Could you check a few things on this model? Use its own coordinates, in mm. A direction names the side the tool comes from. Coordinates: 2 decimals unless noted, no trailing zeros. Loops run counter-clockwise (first coordinate to the right, second up) from the corner with the lowest first, then second, coordinate; pieces in that order, holes last. Notation, with made-up numbers: (80.5, -25.75) - (120.5, -25.75) arc R22 ccw to (120.5, -9.75) - close; hole circle Ø1 at (57, -39). An arc over 180 degrees is marked (long way). One line per item, written item: value. Start each with the question number.
(1) If we section it at A-A on x = 0: Write out the boundary of the cut face in (y, z), then the cut area to 3 significant figures.
(2) If we section it at D-D on z = 15: Write out the boundary of the cut face in (x, y), then the cut area to 3 significant figures.
(3) If we mould it in two halves opening along Y, with no side actions, what happens to faces 4 (the face through (12.932, -5.362, 11.479)), 5 (the face through (-9.5, 0.07, 11.48)), 6 (the face through (2, 5, 39))? For each: pulls with the +Y half, pulls with the -Y half, needs draft (parallel to the pull), parting line crosses it, or undercut.
(4) I'm going to push flat-ended pins straight in: P1, Ø8, axis at x = -5.5, z = 11, coming from the +Y side; P2, Ø5, axis at x = -3.5, z = 8, coming from the +Y side; P3, Ø2, axis at y = 1, z = 12.5, coming from the -X side; P4, Ø3, axis at y = 3, z = 27, coming from the +X side. Where does each tip first touch, or does it pass through?
(5) If we section it at B-B on y = -11: Write out the boundary of the cut face in (x, z), then the cut area to 3 significant figures.
(6) If I drill on line 1 along Y through (x, z) = (0, 10.95); line 2 along Z through (x, y) = (12.5, -4.5); line 3 along Y through (x, z) = (0, 8.5), over which ranges is the centre line in solid material (lowest first)? Write a range as from..to.
(7) On a 3-axis mill with a long thin cutter (end or side, diameter ignored), from which of +Z, -Z, +X, -X, +Y, -Y can I reach the whole of each face in a straight line? I mean faces 1 (the face through (-1.08, -4.88, 2.96)), 2 (the face through (12.5, 0.07, 11.48)), 3 (the face through (-1.08, -4.88, 41.96)). Say none if no direction works.
```python
from build123d import *

# Parameters (mm, degrees)
CROQUIS1_R              = 5
SALIENTE_EXTRUIR1_DEPTH = 6
CROQUIS2_R              = 5.8
SALIENTE_EXTRUIR2_DEPTH = 4
CROQUIS3_R              = 14
SALIENTE_EXTRUIR3_DEPTH = 3
CROQUIS4_R              = 5.8
SALIENTE_EXTRUIR4_DEPTH = 26
CROQUIS5_R              = 5
SALIENTE_EXTRUIR5_DEPTH = 6
CROQUIS6_R              = 1.5
CORTAR_EXTRUIR1_DEPTH   = 6


with BuildPart() as part:
    # Croquis1 → Saliente-Extruir1 (new body)
    with BuildSketch(Plane.XY):
        Circle(CROQUIS1_R)
    extrude(amount=SALIENTE_EXTRUIR1_DEPTH)

    # Croquis2 → Saliente-Extruir2 (add)
    with BuildSketch(Plane.XY.offset(6)):
        Circle(CROQUIS2_R)
    extrude(amount=SALIENTE_EXTRUIR2_DEPTH)

    # Croquis3 → Saliente-Extruir3 (add)
    with BuildSketch(Plane.XY.offset(10)):
        Circle(CROQUIS3_R)
    extrude(amount=SALIENTE_EXTRUIR3_DEPTH)

    # Croquis4 → Saliente-Extruir4 (add)
    with BuildSketch(Plane.XY.offset(13)):
        Circle(CROQUIS4_R)
    extrude(amount=SALIENTE_EXTRUIR4_DEPTH)

    # Croquis5 → Saliente-Extruir5 (add)
    with BuildSketch(Plane.XY.offset(39)):
        Circle(CROQUIS5_R)
    extrude(amount=SALIENTE_EXTRUIR5_DEPTH)

    # Croquis6 → Cortar-Extruir1 (cut)
    with BuildSketch(Plane(origin=(0, 0, 10), x_dir=(-1, 0, 0), z_dir=(0, 0, -1))):
        with Locations((11, 0)):
            Circle(CROQUIS6_R)
        with Locations((0, -11)):
            Circle(CROQUIS6_R)
        with Locations((-11, 0)):
            Circle(CROQUIS6_R)
        with Locations((0, 11)):
            Circle(CROQUIS6_R)
    extrude(amount=-CORTAR_EXTRUIR1_DEPTH, mode=Mode.SUBTRACT)


solid = part.part
```
Values:
1. outline: (-14, 10) - (-12.5, 10) - (-12.5, 13) - (-14, 13) - close; (-9.5, 10) - (-5.8, 10) - (-5.8, 6) - (-5, 6) - (-5, 0) - (5, 0) - (5, 6) - (5.8, 6) - (5.8, 10) - (9.5, 10) - (9.5, 13) - (5.8, 13) - (5.8, 39) - (5, 39) - (5, 45) - (-5, 45) - (-5, 39) - (-5.8, 39) - (-5.8, 13) - (-9.5, 13) - close; (12.5, 10) - (14, 10) - (14, 13) - (12.5, 13) - close
1. area: 534 mm2
2. outline: circle Ø11.6 at (0, 0)
2. area: 106 mm2
3. face 4: parting line crosses it
3. face 5: undercut
3. face 6: needs draft
4. P1: stops at y = 13.92
4. P2: stops at y = 13.86
4. P3: stops at x = -14
4. P4: stops at x = 5.6
5. outline: (-8.66, 10) - (-1.5, 10) - (-1.5, 13) - (-8.66, 13) - close; (1.5, 10) - (8.66, 10) - (8.66, 13) - (1.5, 13) - close
5. area: 43.0 mm2
6. line 1: y = -14..-12.5, -9.5..9.5, 12.5..14
6. line 2: z = 10..13
6. line 3: y = -5.8..5.8
7. face 1: -Z
7. face 2: +Z, -Z
7. face 3: +Z
